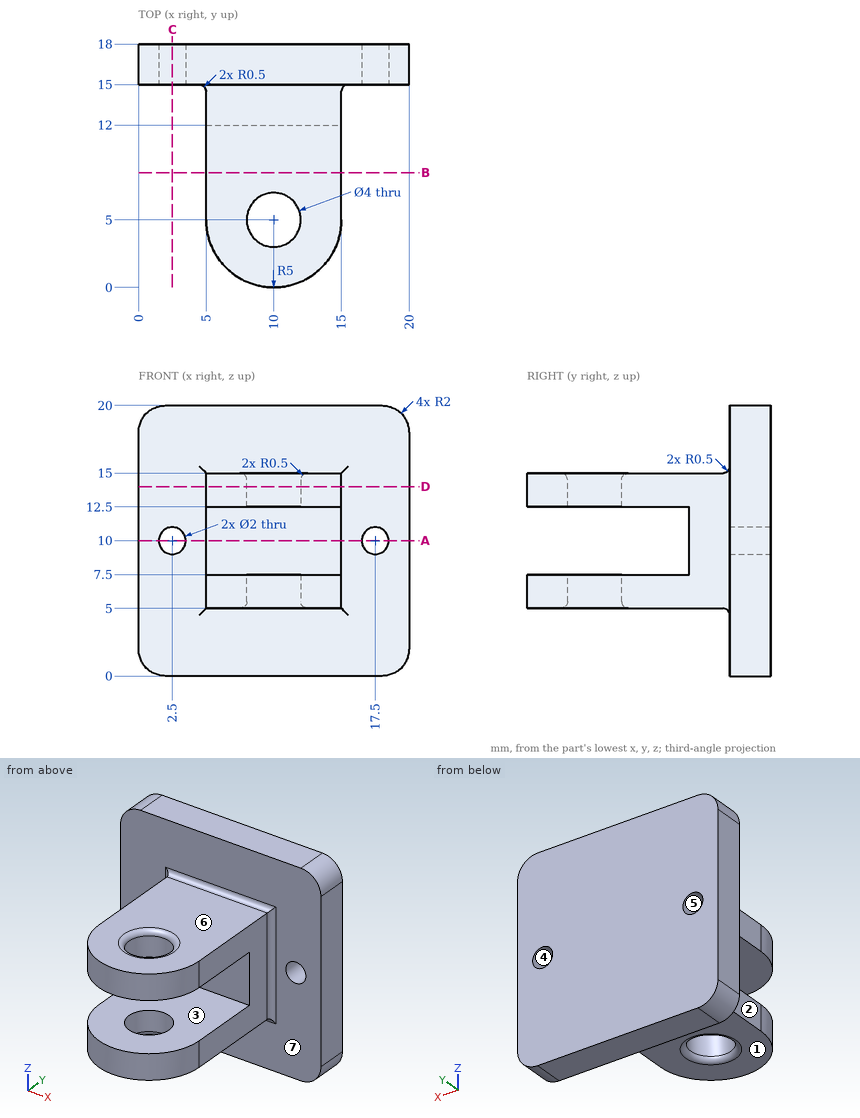
Check sheet for the drawn part. Datum: minimum x, y, z corner. Units: mm. A direction names the side the tool comes from. Round coordinates to 2 decimals unless told otherwise and drop trailing zeros. Write each loop counter-clockwise with the first axis right and the second up, starting at its lowest first coordinate (ties: lowest second). Pieces come first, ordered by that corner, then holes. Notation, with made-up numbers: (0.25, 12) -> (53.25, 12) arc R16 cw to (53.25, 25) -> close; hole circle Ø5 at (10.5, 23). An arc over 180 degrees is marked (long way). One line per item, written item: value. Start each with the question number.
(1) Cross-section at C-C, the plane x = 2.5. Record the cut outline in (y, z).
(2) Cross-section at D-D, the plane z = 14. Record the cut outline in (x, y), and give its area (3 significant figures).
(3) Cross-section at A-A, the plane z = 10. Record the cut outline in (x, y).
(4) Go/stop test with flat-tipped pins: pin 1 Ø4 at (x, z) = (12, 11) entering from -Y; pin 2 Ø8 at (y, z) = (8, 14.5) entering from -X; pin 3 Ø5 at (x, y) = (9, 3.5) entering from -Z; pin 4 Ø3 at (x, y) = (10, 5) entering from +Z. Record where each tip stops, or that it passes through.
(5) Cross-section at B-B, the plane y = 8.5. Record the cut outline in (x, z), and give its area (3 significant figures).
(6) Draft check along Z on the marked faces 4, 5, 6 and 7. Enter one of: +Z half, -Z half, draft (parallel to the pull), parting line (faces both ways), or undercut.
(7) Scan lines: line 1 (X direction, y = 16.2, z = 10); line 2 (Y direction, x = 10, z = 7); line 3 (Z direction, x = 7.75, y = 11). Record each from-to range of solid material in increasing order. Write a range as [from, to].
(8) Access from +Z, -Z, +X, -X, +Y, -Y to the whole of each face (thin tool, end or side, straight path). Record for the marked faces 1, 2 and 3.
Answer:
1. outline: (15, 0) -> (18, 0) -> (18, 9) -> (15, 9) -> close; (15, 11) -> (18, 11) -> (18, 20) -> (15, 20) -> close
2. outline: (0, 15) -> (4.5, 15) arc R0.5 cw to (5, 14.5) -> (5, 5) arc R5 ccw to (15, 5) -> (15, 14.5) arc R0.5 cw to (15.5, 15) -> (20, 15) -> (20, 18) -> (0, 18) -> close; hole circle Ø4 at (10, 5)
2. area: 187 mm²
3. outline: (0, 15) -> (1.5, 15) -> (1.5, 18) -> (0, 18) -> close; (3.5, 15) -> (4.5, 15) arc R0.5 cw to (5, 14.5) -> (5, 12) -> (15, 12) -> (15, 14.5) arc R0.5 cw to (15.5, 15) -> (16.5, 15) -> (16.5, 18) -> (3.5, 18) -> close; (18.5, 15) -> (20, 15) -> (20, 18) -> (18.5, 18) -> close
4. pin 1: y = 0.05
4. pin 2: x = 5
4. pin 3: z = 5
4. pin 4: through
5. outline: (5, 5) -> (15, 5) -> (15, 7.5) -> (5, 7.5) -> close; (5, 12.5) -> (15, 12.5) -> (15, 15) -> (5, 15) -> close
5. area: 50.0 mm²
6. face 4: undercut
6. face 5: undercut
6. face 6: +Z half
6. face 7: draft
7. line 1: [0, 1.5], [3.5, 16.5], [18.5, 20]
7. line 2: [0, 3], [7, 18]
7. line 3: [5, 7.5], [12.5, 15]
8. face 1: -Z, +X, -X, -Y
8. face 2: +Z, -Z, -X, -Y
8. face 3: +X, -X, -Y
